Model file for the job. Use its own axes, mm. A direction names the side the tool comes from. Coordinates: 2 decimals unless noted, no trailing zeros. Write each loop counter-clockwise with the first axis right and the second up, starting at its lowest first coordinate (ties: lowest second). Pieces come first, ordered by that corner, then holes. Notation, with made-up numbers: (-2, 81) - (9, 81) arc R6 cw to (9, 85) - close; hole circle Ø6 at (18, 74.25). An arc over 180 degrees is marked (long way). Put each result on its own line as item: value. Start each with the question number.
1. Pull direction Y, two halves, no side cores. Call faces 1 (the face through (2, -20, -40)), 2 (the face through (2, -40, -11)), 3 (the face through (2, -12.275, 38)), 4 (the face through (2, -5, -36.825)): released by +Y, released by -Y, zero draft, split by the parting line, or undercut.
2. Saw through at B-B, the plane y = 25. Write the cut outline in (x, z) (3 decimals).
3. Which spindle directions (+Z, -Z, +X, -X, +Y, -Y) get a long thin tool onto all of the face, cutting with end or side? Do faces 5 (the face through (2, -36.825, -5)), 6 (the face through (2, -34, -36.825)), 7 (the face through (2, 22.095, -38)), 8 (the face through (2, 36.825, -16)), 9 (the face through (2, -34, 36.825)). Say none if no direction does.
4. Drill centre lines: L1, parallel to Z at x = 2.8, y = -26 (3 decimals); L2, parallel to Z at x = 1.9, y = 5.5 (3 decimals). Where is each one in solid material? Low to high. Write a range as from..to.
5. Drop flat-ended pins along their axis: P1, Ø10, axis at y = -23.5, z = 13, coming from the -X side; P2, Ø1.6, axis at x = 2, y = -38, coming from the -Z side; P3, Ø1.6, axis at x = 1, y = -38, coming from the +Z side; P4, Ø1.6, axis at x = 2.5, z = -39, coming from the +Y side (3 decimals). Give the stop position or say it passes through.
6. Saw through at A-A, the plane z = 16. Write the cut outline in (x, y) (3 decimals).
```python
from build123d import *

# Parameters (mm, degrees)
SKETCH2_W           = 80
SKETCH2_H           = 80
BOSS_EXTRUDE1_DEPTH = 3.175
SKETCH3_OUTSIDE_W   = 104.636
SKETCH3_OUTSIDE_H   = 104.636
CUT_EXTRUDE1_DEPTH  = 57.657573413
SKETCH5_W           = 3.175000001
SKETCH5_H           = 44.189999998
BOSS_EXTRUDE3_DEPTH = 3.175


with BuildPart() as part:
    # Sketch2 → Boss-Extrude1 (new body)
    with BuildSketch(Plane(origin=(0, 0, 0), x_dir=(0, 0, -1), z_dir=(1, 0, 0))):
        Rectangle(SKETCH2_W, SKETCH2_H)
    extrude(amount=BOSS_EXTRUDE1_DEPTH)

    # Sketch3 outside → Cut-Extrude1 (cut, through all)
    with BuildSketch(Plane(origin=(3.175, 0, 0), x_dir=(0, 0, -1), z_dir=(1, 0, 0))):
        Rectangle(SKETCH3_OUTSIDE_W, SKETCH3_OUTSIDE_H)
        Polygon((-36.824999999, 36.825), (-34.666666667, 36.824999997), (-34.666666667, 39.999999997), (-29.333333333, 39.999999997), (-29.333333333, 36.824999997), (-24, 36.824999997), (-24, 40), (-18.666666667, 40), (-18.666666667, 36.825), (-13.333333333, 36.825), (-13.333333333, 40), (-8, 40), (-8, 36.825), (-2.666666667, 36.825), (-2.666666667, 40), (2.666666667, 40), (2.666666667, 36.825), (8, 36.825), (8, 40), (13.333333333, 40), (13.333333333, 36.825), (18.666666667, 36.825), (18.666666667, 40), (24, 40), (24, 36.825), (29.333333333, 36.825), (29.333333333, 40), (34.666666667, 40), (34.666666667, 36.825), (36.824999999, 36.825), (36.824999999, 31.915), (40, 31.915000001), (40, 27.005), (36.824999999, 27.005), (36.824999999, 22.095000001), (40, 22.095000001), (40, 17.185000001), (36.824999999, 17.185000001), (36.824999999, 12.275000001), (40, 12.275000001), (40, 7.365000001), (36.824999999, 7.365000001), (36.824999999, 2.455000001), (40, 2.455000002), (40, -2.454999999), (36.824999999, -2.454999999), (36.824999999, -7.364999998), (40, -7.364999998), (40, -12.274999998), (36.824999999, -12.274999998), (36.824999999, -17.184999998), (40, -17.184999998), (40, -22.094999998), (36.824999999, -22.094999998), (36.824999999, -27.004999998), (40, -27.004999997), (40, -31.914999997), (36.824999999, -31.914999997), (36.824999999, -36.824999997), (34.666666667, -36.825), (34.666666667, -40), (29.333333333, -40), (29.333333333, -36.825), (24, -36.825), (24, -40), (18.666666667, -40), (18.666666667, -36.825), (13.333333333, -36.825), (13.333333333, -40), (8, -40), (8, -36.825), (2.666666667, -36.825), (2.666666667, -40), (-2.666666667, -40), (-2.666666667, -36.825), (-8, -36.825), (-8, -40), (-13.333333333, -40), (-13.333333333, -36.825), (-18.666666667, -36.825), (-18.666666667, -40), (-24, -40), (-24, -36.824999997), (-29.333333333, -36.824999997), (-29.333333333, -39.999999997), (-34.666666667, -39.999999997), (-34.666666667, -36.824999997), (-36.825, -36.824999997), (-36.825, -31.914999997), (-40.000000001, -31.914999997), (-40.000000001, -27.004999997), (-36.825, -27.004999997), (-36.825, -22.094999998), (-40.000000001, -22.094999997), (-40.000000001, -17.184999998), (-36.825, -17.184999998), (-36.825, -12.274999998), (-40.000000001, -12.274999998), (-40, -7.364999998), (-36.825, -7.364999998), (-36.825, -2.454999999), (-40, -2.454999998), (-40, 2.455000002), (-36.825, 2.455000002), (-36.825, 7.365000001), (-40, 7.365000002), (-40, 12.275000001), (-36.825, 12.275000001), (-36.824999999, 17.185000001), (-40, 17.185000002), (-40, 22.095000001), (-36.824999999, 22.095000001), (-36.824999999, 27.005000001), (-40, 27.005000001), (-40, 31.915000001), (-36.824999999, 31.915000001), align=None, mode=Mode.SUBTRACT)
    extrude(amount=-CUT_EXTRUDE1_DEPTH, mode=Mode.SUBTRACT)

    # Sketch5 → Boss-Extrude3 (add)
    with BuildSketch(Plane.ZY):
        with Locations((38.412499999, 14.730000001)):
            Rectangle(SKETCH5_W, SKETCH5_H)
    extrude(amount=-BOSS_EXTRUDE3_DEPTH)


solid = part.part
```
Final values:
1. face 1: zero draft
1. face 2: released by -Y
1. face 3: undercut
1. face 4: undercut
2. outline: (0, -36.825) - (3.175, -36.825) - (3.175, 40) - (0, 40) - close
3. face 5: +X, -X, -Y
3. face 6: -Z, +X, -X, -Y
3. face 7: -Z, +X, -X
3. face 8: +X, -X, +Y
3. face 9: +Z, +X, -X, -Y
4. L1: z = -36.825..36.825
4. L2: z = -36.825..40
5. P1: stops at x = 0
5. P2: stops at z = -34.67
5. P3: stops at z = 34.67
5. P4: stops at y = 31.915
6. outline: (0, -36.825) - (3.175, -36.825) - (3.175, 36.825) - (0, 36.825) - close
